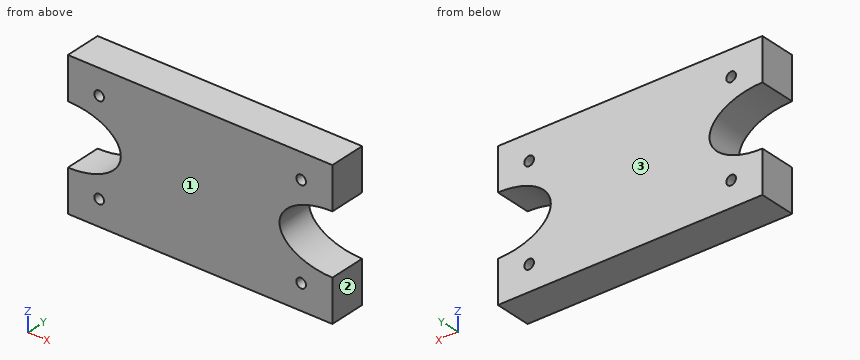
```python
from build123d import *

# Parameters (mm, degrees)
ESQUISSE1_W             = 110
ESQUISSE1_H             = 60
BOSS_EXTRU_1_DEPTH      = 15.3
ESQUISSE2_R             = 2
ENL_V_MAT_EXTRU_2_DEPTH = 87.616374477
ESQUISSE5_RX            = 22
ESQUISSE5_RY            = 12.5
ENL_V_MAT_EXTRU_4_DEPTH = 87.616374477


with BuildPart() as part:
    # Esquisse1 → Boss.-Extru.1 (new body)
    with BuildSketch(Plane(origin=(0, 0, 0), x_dir=(1, 0, 0), z_dir=(0, 1, 0))):
        with Locations((19.731995919, -11.029685758)):
            Rectangle(ESQUISSE1_W, ESQUISSE1_H)
    extrude(amount=BOSS_EXTRU_1_DEPTH)

    # Esquisse2 → Enlèv. mat.-Extru.2 (cut, through all)
    with BuildSketch(Plane(origin=(0, 15.3, 0), x_dir=(1, 0, 0), z_dir=(0, 1, 0))):
        with Locations(Location((61.731995919, 8.470314242, 0), (0, 0, 270))):
            Circle(ESQUISSE2_R)
        with Locations(Location((61.731995919, -30.529685758, 0), (0, 0, 270))):
            Circle(ESQUISSE2_R)
        with Locations(Location((-22.268004081, 8.470314242, 0), (0, 0, 270))):
            Circle(ESQUISSE2_R)
        with Locations(Location((-22.268004081, -30.529685758, 0), (0, 0, 270))):
            Circle(ESQUISSE2_R)
    extrude(amount=-ENL_V_MAT_EXTRU_2_DEPTH, mode=Mode.SUBTRACT)

    # Esquisse5 → Enlèv. mat.-Extru.4 (cut, through all)
    with BuildSketch(Plane(origin=(0, 15.3, 0), x_dir=(1, 0, 0), z_dir=(0, 1, 0))):
        with Locations((-35.268004081, -11.029685758)):
            Ellipse(ESQUISSE5_RX, ESQUISSE5_RY)
        with Locations(Location((74.731995919, -11.029685758), (0, 0, 180))):
            Ellipse(ESQUISSE5_RX, ESQUISSE5_RY)
    extrude(amount=-ENL_V_MAT_EXTRU_4_DEPTH, mode=Mode.SUBTRACT)


solid = part.part
```
Model file for the job. Use its own axes, mm. Face numbers are marked on the shaded views. Coordinates: 2 decimals unless noted, no trailing zeros. Loops run counter-clockwise (first coordinate to the right, second up) from the corner with the lowest first, then second, coordinate; pieces in that order, holes last. Notation, with made-up numbers: M 16,-16.5 L 67,-16.5 A21 cw 67,-2.5 Z; hole C 73,89.5 d10. An arc over 180 degrees is marked long. Use CSV: the item, a comma, the result in double quotes. Start each with the question number.
1. Band-saw the part on B-B, the plane y = 4.25. Give the number of separate pieces and of enclosed holes in the cut face, then the cut area to 3 significant figures.
2. Probe probe 1 along X at (y, z) = (1.25, 31); probe 2 along Z at (x, y) = (63.5, 10.75); probe 3 along X at (y, z) = (4, 10.5). List the from-to ranges inside material, lowest first. Write a range as [from, to].
3. Band-saw the part on A-A, the plane z = 30. List the corners of the cut face in (x, y).
4. Two-plate mould, pull along Y, no slides. Class the marked faces 1, 2 and 3: pulls with the +Y half, pulls with the -Y half, needs draft (parallel to the pull), parting line crosses it, or undercut.
5. Flat gauge pins, fed straight in: pin 1 (5 mm diameter, centred on x = -22.27, z = 30.53, fed in from +Y); pin 2 (2.5 mm diameter, centred on x = 61.73, z = 30.53, fed in from -Y). Where does each tip first touch, or does it go through?
Entries:
1,separate pieces,"1"
1,enclosed holes,"4"
1,area,"5,690 mm2"
2,probe 1,"x = [-35.27, -24.21], [-20.32, 59.79], [63.68, 74.73]"
2,probe 2,"z = [-18.97, -9.41], [-7.54, 0.28], [21.78, 29.59], [31.46, 41.03]"
2,probe 3,"x = [-13.29, 52.75]"
3,outline,"M -35.27,0 L -24.2,0 L -24.2,15.3 L -35.27,15.3 Z; M -20.34,0 L 59.8,0 L 59.8,15.3 L -20.34,15.3 Z; M 63.66,0 L 74.73,0 L 74.73,15.3 L 63.66,15.3 Z"
4,face 1,"pulls with the -Y half"
4,face 2,"needs draft"
4,face 3,"pulls with the +Y half"
5,pin 1,"stops at y = 15.3"
5,pin 2,"passes through"
